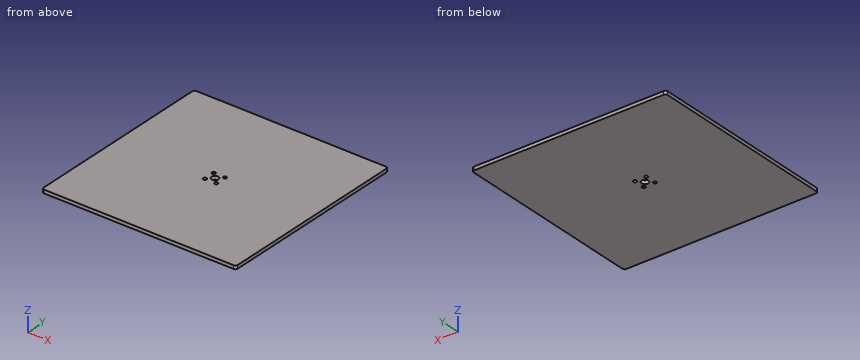
```python
from build123d import *

# Parameters (mm, degrees)
SKETCH_1_W          = 170
SKETCH_1_H          = 170
EXTRUDE_1_DEPTH     = 3
SKETCH_3_R          = 3
SKETCH_3_R_2        = 1.5
CUT_EXTRUDE_1_DEPTH = 121.245582039
FILLET_1_R          = 2


with BuildPart() as part:
    # 草图1 → 凸台-拉伸1 (new body)
    with BuildSketch(Plane.XY):
        Rectangle(SKETCH_1_W, SKETCH_1_H)
    extrude(amount=EXTRUDE_1_DEPTH)

    # 草图3 → 切除-拉伸1 (cut, through all)
    with BuildSketch(Plane(origin=(0, 0, 0), x_dir=(-1, 0, 0), z_dir=(0, 0, -1))):
        Circle(SKETCH_3_R)
        with Locations((4.95, 4.95)):
            Circle(SKETCH_3_R_2)
        with Locations((-4.95, 4.95)):
            Circle(SKETCH_3_R_2)
        with Locations((-4.95, -4.95)):
            Circle(SKETCH_3_R_2)
        with Locations((4.95, -4.95)):
            Circle(SKETCH_3_R_2)
    extrude(amount=-CUT_EXTRUDE_1_DEPTH, mode=Mode.SUBTRACT)

    # 圆角1
    fillet_1_edges = [part.edges().sort_by_distance(p)[0] for p in [
        (-85, 85, 1.5),
        (85, 85, 1.5),
        (85, -85, 1.5),
        (-85, -85, 1.5),
    ]]
    fillet(fillet_1_edges, radius=FILLET_1_R)


solid = part.part
```
Could you check a few things on this model? Use its own coordinates, in mm. Round coordinates to 2 decimals unless told otherwise and drop trailing zeros. Loops run counter-clockwise (first coordinate to the right, second up) from the corner with the lowest first, then second, coordinate; pieces in that order, holes last.
Q1. I want a section at A-A (y = 0). Write out the boundary of the cut face in (x, z).
Q2. Please list where these lines run through material, in increasing order: L1, parallel to Y at x = -4.95, z = 2.4; L2, parallel to Y at x = 0, z = 0.6.
Answer below:
1. outline: (-85, 0) - (-3, 0) - (-3, 3) - (-85, 3) - close; (3, 0) - (85, 0) - (85, 3) - (3, 3) - close
2. L1: y = -85 to -6.45, -3.45 to 3.45, 6.45 to 85
2. L2: y = -85 to -3, 3 to 85
